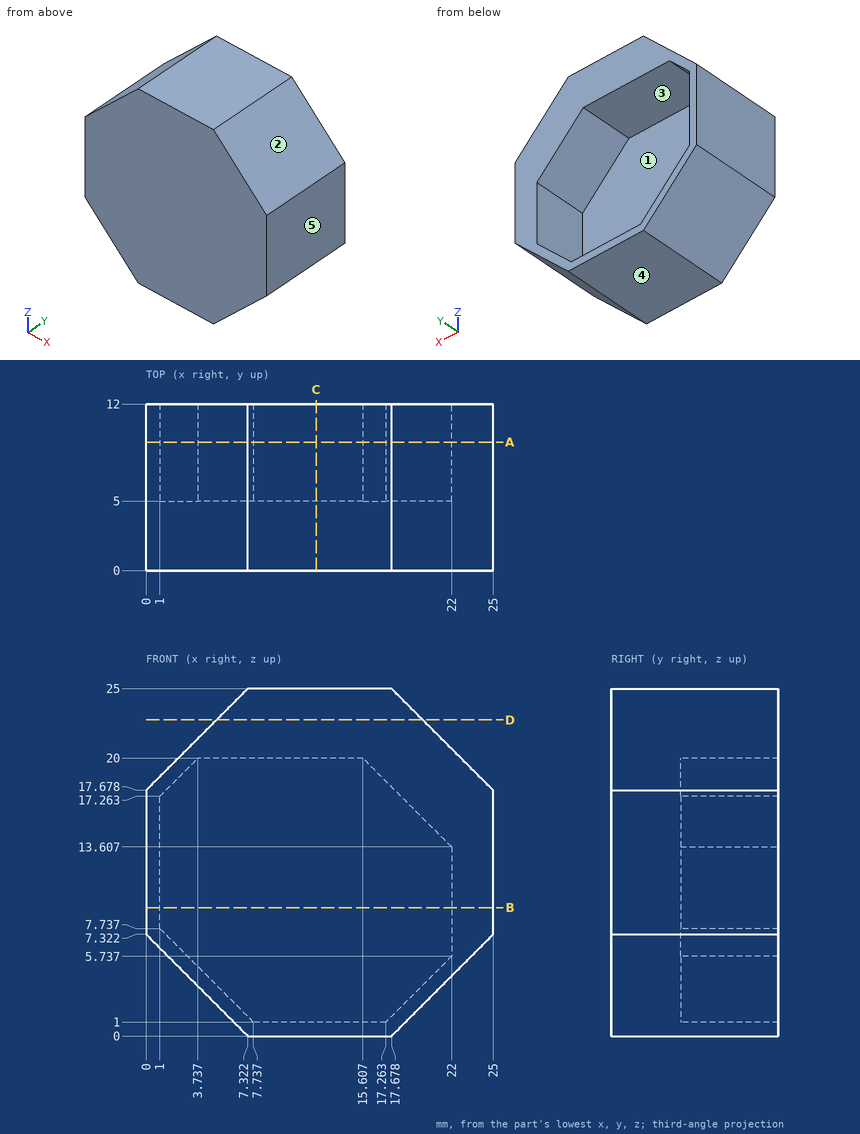
Study the drawing (mm; zero at the part's minimum x, y, z) and answer. A direction names the side the tool comes from. Round coordinates to 2 decimals unless told otherwise and drop trailing zeros. Loops run counter-clockwise (first coordinate to the right, second up) from the corner with the lowest first, then second, coordinate; pieces in that order, holes last. Notation, with made-up numbers: (7.25, -19) -> (55.25, -19) arc R18 cw to (55.25, 14) -> close; hole circle Ø1 at (50.5, 81). An arc over 180 degrees is marked (long way). Write each question's results on one line, items separated by ' | '. Start each with the question number.
1. Section B-B (z = 9.25) is taken. Determine the outline of the cut face in (x, y), plus the area to 3 significant figures.
2. Section A-A (y = 9.25) is taken. Determine the outline of the cut face in (x, z), plus the area to 3 significant figures.
3. A tool of negligible diameter and unlimited length cuts with its end or side. For the marked faces 1 and 2, from which of +Z, -Z, +X, -X, +Y, -Y can it reach the whole face along a straight path? Write none if from no direction.
4. For a pull along Z with two mould halves and no side action, classify the marked faces 3, 4 and 5 as +Z half, -Z half, draft (parallel to the pull), parting line (faces both ways), or undercut.
5. Section C-C (x = 12.25) is taken. Determine the outline of the cut face in (y, z).
6. Find the intervals of material crossed by probe 1 along Z at (x, y) = (11, 7); probe 2 along X at (y, z) = (10, 13); probe 3 along Y at (x, z) = (16.75, 6.75), in increasing order. Write a range as from..to.
7. Given pin 1 Ø10 at (x, z) = (16, 9) entering from +Y; pin 2 Ø2 at (x, y) = (22, 8) entering from +Z, each flat-ended and moving along its own axis, determine where each tip first touches the part or whether it passes through.
8. Section D-D (z = 22.75) is taken. Determine the outline of the cut face in (x, y), plus the area to 3 significant figures.
Evaluation:
1) outline: (0, 0) -> (25, 0) -> (25, 12) -> (22, 12) -> (22, 5) -> (1, 5) -> (1, 12) -> (0, 12) -> close | area: 153 mm2
2) outline: (0, 7.32) -> (7.32, 0) -> (17.68, 0) -> (25, 7.32) -> (25, 17.68) -> (17.68, 25) -> (7.32, 25) -> (0, 17.68) -> close; hole (1, 7.74) -> (7.74, 1) -> (17.26, 1) -> (22, 5.74) -> (22, 13.61) -> (15.61, 20) -> (3.74, 20) -> (1, 17.26) -> close | area: 177 mm2
3) face 1: +Y | face 2: +Z, +X, +Y, -Y
4) face 3: undercut | face 4: -Z half | face 5: draft
5) outline: (0, 0) -> (12, 0) -> (12, 1) -> (5, 1) -> (5, 20) -> (12, 20) -> (12, 25) -> (0, 25) -> close
6) probe 1: z = 0..1, 20..25 | probe 2: x = 0..1, 22..25 | probe 3: y = 0..5
7) pin 1: stops at y = 5 | pin 2: stops at z = 21.68
8) outline: (5.07, 0) -> (19.93, 0) -> (19.93, 12) -> (5.07, 12) -> close | area: 178 mm2
